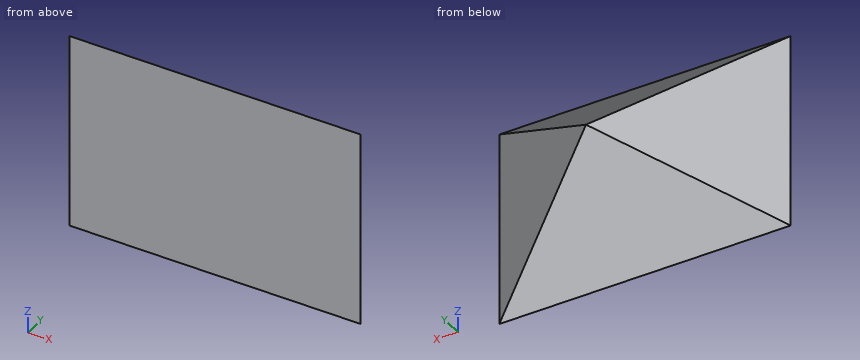
from build123d import *

# Parameters (mm, degrees)
AUFSATZ_LINEAR_START            = -68.111592
SKIZZE5_W                       = 2000
SKIZZE5_H                       = 1500
AUFSATZ_LINEAR_AUSTRAGEN1_DEPTH = 63.5
HORIZONTAL_DEPTH                = 1501
VERTIKAL_DEPTH                  = 78.537939311
VERTIKAL_DEPTH_BACK             = 78.537939311


with BuildPart() as part:
    # Skizze5 → Aufsatz-Linear austragen1 (new body)
    with BuildSketch(Plane(origin=(0, 0, 0), x_dir=(1, 0, 0), z_dir=(0, 1, 0)).offset(AUFSATZ_LINEAR_START)):
        Rectangle(SKIZZE5_W, SKIZZE5_H)
    extrude(amount=AUFSATZ_LINEAR_AUSTRAGEN1_DEPTH)

    # Skizze6 → Horizontal (cut, through all)
    with BuildSketch(Plane.XY.offset(750)):
        Polygon((0, -15.811591556), (-1000, -690.320108399), (-1000, -3.611591556), (1000, -3.611591556), (1000, -690.320108399), align=None)
    extrude(amount=-HORIZONTAL_DEPTH, mode=Mode.SUBTRACT)

    # Skizze7 → Vertikal (cut, two sides)
    with BuildSketch(Plane.ZY) as vertikal_sk:
        Polygon((0, -15.811591556), (-750, -765.811591556), (-750, -14.811591556), (750, -14.811591556), (750, -765.811591556), align=None)
    extrude(amount=VERTIKAL_DEPTH, mode=Mode.SUBTRACT)
    extrude(vertikal_sk.sketch, amount=-VERTIKAL_DEPTH_BACK, mode=Mode.SUBTRACT)


solid = part.part
For this review, take the finished solid that the model builds, in its own axes (mm). Round coordinates to 2 decimals unless told otherwise and drop trailing zeros. Order: outer loops, then holes, each group sorted by start corner. A loop starts at its lowest first (then second) coordinate and runs counter-clockwise, first axis right, second up. Notation, with made-up numbers: (68, 84) -> (82, 84) arc R28 cw to (82, 123) -> close; hole circle Ø11 at (54.5, 57). An arc over 180 degrees is marked (long way). Put each result on its own line as item: value.
Q1. Add section B-B on z = -10.5. Write out the cut boundary in (x, y), plus the area to 3 significant figures.
Check result:
outline: (-77.54, -68.11) -> (77.54, -68.11) -> (15.57, -26.31) -> (-15.57, -26.31) -> close
area: 3,890 mm2
Q2. Add section A-A on x = -65.5. Write out the cut boundary in (y, z), plus the area to 3 significant figures.
Check result:
outline: (-68.11, -52.3) -> (-59.99, -44.18) -> (-59.99, 44.18) -> (-68.11, 52.3) -> close
area: 783 mm2
Q3. For probe 1 along Y at (x, z) = (-57, -2); probe 2 along X at (y, z) = (-44, 7); probe 3 along X at (y, z) = (-41, -9), list the stretches that pass through material, from the lowest coordinate up. Write a range as [from, to].
Check result:
probe 1: [-68.11, -54.26]
probe 2: [-41.79, 41.79]
probe 3: [-37.34, 37.34]
Q4. Insertion check: pin 1 Ø10 at (y, z) = (-30, 13) entering from -X; pin 2 Ø4 at (x, y) = (59, -54.5) entering from -Z; pin 3 Ø4 at (x, z) = (1.5, 32) entering from +Y. Each pin has a flat end and moves straight along its axis. Give the tip position at first contact, or say it passes through.
Check result:
pin 1: x = -28.45
pin 2: z = -40.69
pin 3: y = -45.81
